For this review, take the finished solid that the model builds, in its own axes (mm). Face numbers are marked on the shaded views. A direction names the side the tool comes from. Coordinates: 2 decimals unless noted, no trailing zeros. Loops run counter-clockwise (first coordinate to the right, second up) from the corner with the lowest first, then second, coordinate; pieces in that order, holes last. Notation, with made-up numbers: M -16.75,-28 L 40.25,-28 A9 cw 40.25,-21 Z; hole C 1,73.25 d11. An arc over 180 degrees is marked long. Answer as a JSON object with one key per item and string values. Group by question number.
Item 1: Wall thickness on L1, parallel to Y at x = 0.5, z = 9; L2, parallel to Z at x = 18, y = -1.5; L3, parallel to Y at x = 40.5, z = 4.5: over which ranges is each line inside the solid? List them lowest first. Write a range as from..to.
Item 2: Mouldability with a two-part tool opening along X and no side actions: class the marked faces 1, 2 and 3 as +X half, -X half, draft (parallel to the pull), parting line (faces both ways), or undercut.
Item 3: Add section A-A (y = 0). Count the separate pieces of the cut face and the enclosed holes in it, then the cut area to 3 significant figures.
Item 4: Add section D-D (x = 37.5). State the section outline as (y, z) points.
Item 5: Insertion check: pin 1 (3 mm diameter, centred on x = 29.16, y = -29.16, fed in from -Z); pin 2 (2 mm diameter, centred on x = 29.16, y = 29.16, fed in from -Z); pin 3 (1 mm diameter, centred on x = -12.5, z = 2.5, fed in from +Y); pin 4 (3 mm diameter, centred on x = 19.5, z = 9, fed in from +Y). Each pin has a flat end and moves straight along its axis. Give the tip position at first contact, or say it passes through.
Item 6: Add section C-C (x = 3). State the section outline as (y, z) points.
Item 7: Tool access review of the marked faces 4, 5 and 6: name each direction out of +Z, -Z, +X, -X, +Y, -Y from which nothing blocks a thin tool from reaching the whole face with its end or side.
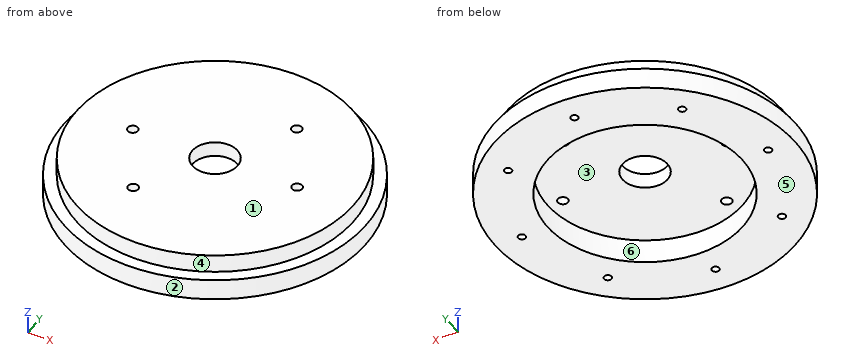
Autodesk Inventor part; units mm, degrees
ref_plane "Work Plane1" through (0, 0, 22) normal (0, 0, 1) x (1, 0, 0)
ref_plane "Plano de trabajo2" through (0, 0, 54) normal (0, 0, 1) x (1, 0, 0)
ref_plane "YZ Plane" through (0, 0, 0) normal (1, 0, 0) x (0, 1, 0)
sketch "Sketch1" plane through (0, 0, 0) normal (0, 0, 1) x (1, 0, 0)
  circle A0 centre (0, 0) radius 50
  circle A1 centre (0, 0) radius 12.5
  circle A2 centre (0, 0) radius 14.5
  line L0 (-15.5, -15.5) -> (15.5, -15.5) construction
  line L1 (15.5, -15.5) -> (15.5, 15.5) construction
  line L2 (15.5, 15.5) -> (-15.5, 15.5) construction
  line L3 (-15.5, 15.5) -> (-15.5, -15.5) construction
  line L4 (-15.5, -15.5) -> (15.5, 15.5) construction
  line L5 (15.5, -15.5) -> (-15.5, 15.5) construction
  dimension "Diametro" = 100
  dimension "d1" = 25
  dimension "d2" = 2
  dimension "d8" = 31
extrude "Extrusion1" add sketch "Sketch1" along normal blind 7 contours A0 | A2
extrude "Extrusion2" add sketch "Sketch1" along normal blind 100 contours A2
ref_plane "Work Plane1" through (0, 0, 22) normal (0, 0, 1) x (1, 0, 0)
sketch "Sketch2" plane through (0, 0, 22) normal (0, 0, 1) x (1, 0, 0)
  arc A0 (2.5, 24.8747) -> (-2.5, 24.8747) centre (0, 0) ccw
  line L0 (2.5, 24.8747) -> (2.5, 14.2829)
  line L1 (-2.5, 24.8747) -> (-2.5, 14.2829)
  line L2 (0, -70) -> (0, 70)
  circle A1 centre (0, 0) radius 14.5
  point P0 (0, 25)
  dimension "d24" = 5
  dimension "d25" = 25
  dimension "Dedos" = 5
extrude "Extrusion3" add sketch "Sketch2" along normal blind 15 contours L0 A1 L2 A0 | L2 A1 L1 A0
sketch "Sketch3" plane through (0, 0, 0) normal (1, 0, 0) x (0, 1, 0)
  line L0 (25, 37) -> (24.8747, 37)
  line L1 (14.2829, 22) -> (14.5, 22)
  line L2 (25, 22) -> (25, 37)
  line L3 (14.2829, 22) -> (14.2829, 37)
  circle A0 centre (25.74, 29.5) radius 1.5
  line L4 (0, -7.4) -> (0, 44.4)
  point P0 (0, 0)
  point P1 (25, 29.5)
  dimension "d31" = 3
  dimension "d92" = 25.74
fillet "Fillet2" radius 8 1 edges at (0, 25, 22)
pattern_circular "Circular Pattern1" count 4 over 360 about axis through (0, 0, 0) along (0, 0, 1) of "Fillet2", "Extrusion3"
ref_plane "Plano de trabajo2" through (0, 0, 54) normal (0, 0, 1) x (1, 0, 0)
sketch "Boceto4" plane through (0, 0, 54) normal (0, 0, 1) x (1, 0, 0)
  circle A0 centre (0, 0) radius 17.5
  circle A1 centre (0, 0) radius 14.5
  line L0 (4, -23.75) -> (4, -26.75)
  dimension "d54" = 35
extrude "Extrusión5" add sketch "Boceto4" against normal up to surface (47 mm away)
sketch "Boceto5" plane through (0, 0, 37) normal (0, 0, 1) x (0, 1, 0)
  arc A0 (-2.5, -17.3205) -> (2.5, -17.3205) centre (0, 0) ccw
  line L0 (-2.5, -17.3205) -> (-2.5, -24.8747)
  arc A1 (-2.5, -24.8747) -> (2.5, -24.8747) centre (0, 0) ccw
  line L1 (2.5, -24.8747) -> (2.5, -17.3205)
  circle A2 centre (0, 0) radius 14.5
  line L2 (2.5, -17.3205) -> (2.5, -14.2829)
  line L3 (-2.5, -17.3205) -> (-2.5, -14.2829)
extrude "Extrusión6" add sketch "Boceto5" along normal blind 20 contours L3 A2 L2 A0 | A0 L1 A1 L0
fillet "Empalme4" radius 8 1 edges at (25, 0, 57)
pattern_circular "Patrón circular2" count 4 over 360 about axis through (0, 0, 54) along (0, 0, -1) of "Extrusión6", "Empalme4"
chamfer "Chaflán1" distance 2 angle 45 1 edges at (-14.5, 0, 100)
sketch "Boceto6" plane through (0, 0, 7) normal (0, 0, 1) x (1, 0, 0)
  circle A0 centre (0, 0) radius 50
  arc A1 (17.3205, 2.5) -> (2.5, 17.3205) centre (0, 0) ccw construction
  line L0 (0, 0) -> (32.476, 18.75) construction
  arc A2 (17.3205, 2.5) -> (2.5, 17.3205) centre (0, 0) ccw construction
  point P0 (16.25, -6.4952)
  point P1 (16.25, 6.4952)
  point P2 (0, 37.5)
  point P3 (-32.476, 18.75)
  point P4 (-32.476, -18.75)
  point P5 (0, -37.5)
  point P6 (32.476, -18.75)
  point P7 (10.8253, 13.75)
  point P8 (15.1554, 8.75)
  dimension "d73" = 360
  dimension "d91" = 37.5
sketch "Boceto8" plane through (0, 0, 7) normal (0, 0, 1) x (1, 0, 0)
  circle A0 centre (0, 0) radius 17.5
  circle A1 centre (0, 0) radius 50
  circle A2 centre (0, 0) radius 46
  dimension "Espesor" = 4
extrude "Extrusión8" add sketch "Boceto8" along normal blind 6 contours A2
sketch "Boceto9" plane through (2.5, 14.0104, 54) normal (1, 0, 0) x (0, -1, 0)
  line L0 (16.5104, 0) -> (28.2932, 0)
  line L1 (-35.9896, 54) -> (64.0104, 54)
  point P0 (1.4018, 24.5)
  point P1 (22.4018, 0)
  dimension "d124" = 21
  dimension "d125" = 29.5
hole "Agujero4" at (2.5, 12.6086, 29.5) direction (-1, 0, 0) diameter 3.4 depth 5
pattern_circular "Patrón circular3" count 4 over 360 about axis through (0, 0, 54) along (0, 0, -1) of "Agujero4"
sketch "Boceto13" plane through (0, 0, 13) normal (0, 0, 1) x (1, 0, 0)
  point P0 (0, 0)
sketch "Boceto15" plane through (0, 0, 0) normal (0, 0, -1) x (-1, 0, 0)
  circle A0 centre (0, 0) radius 27.5 construction
  point P0 (27.5, 0)
  point P1 (13.75, 23.8157)
  point P2 (-13.75, 23.8157)
  point P3 (-27.5, 0)
  point P4 (-13.75, -23.8157)
  point P5 (13.75, -23.8157)
  dimension "d134" = 55
  dimension "d137" = 360
hole "Agujero8" at (-13.75, -23.8157, 0) at (13.75, -23.8157, 0) at (27.5, 0, 0) at (13.75, 23.8157, 0) at (-13.75, 23.8157, 0) at (-27.5, 0, 0) direction (0, 0, 1) diameter 3.4 end through all
sketch "Boceto16" plane through (0, 0, 0) normal (0, 0, -1) x (-1, 0, 0)
  circle A0 centre (0, 0) radius 32.465
  dimension "d146" = 64.93
extrude "Extrusión10" cut sketch "Boceto16" against normal blind 8
sketch "Boceto18" plane through (0, 0, 0) normal (0, 0, -1) x (-1, 0, 0)
  point P0 (0, 0)
  point P1 (-41.233, 0)
  point P2 (-29.1561, -29.1561)
  point P3 (0, -41.233)
  point P4 (29.1561, -29.1561)
  point P5 (41.233, 0)
  point P6 (29.1561, 29.1561)
  point P7 (0, 41.233)
  point P8 (-29.1561, 29.1561)
  dimension "d162" = 41.233
  dimension "d165" = 360
hole "Agujero10" at (41.233, 0, 0) at (29.1561, -29.1561, 0) at (0, -41.233, 0) at (-29.1561, -29.1561, 0) at (-41.233, 0, 0) at (-29.1561, 29.1561, 0) at (0, 41.233, 0) at (29.1561, 29.1561, 0) direction (0, 0, 1) diameter 2.459 depth 10
sketch "Sketch19" plane through (14.2829, -2.5, 54) normal (0, -1, 0) x (1, 0, 0)
  circle A0 centre (6.7167, -24.5) radius 1.7
  line L0 (3.0377, 0) -> (3.0377, -31.9844)
  line L1 (3.0377, 0) -> (-11.7829, 0)
  point P0 (-14.2829, -54)
  dimension "d174" = 3.4
  dimension "d175" = 3.679
  dimension "d176" = 24.5
hole "Hole11" at (20.9995, -2.5, 29.5) direction (0, 1, 0) diameter 4 depth 5
pattern_circular "Circular Pattern4" count 4 over 360 about axis through (0, 0, 0) along (0, 0, 1) of "Hole11"
sketch "Sketch20" plane through (0, 0, 13) normal (0, 0, 1) x (1, 0, 0)
  circle A0 centre (-27.5, 0) radius 1.7
  circle A1 centre (-13.75, 23.8157) radius 1.7
  circle A2 centre (13.75, 23.8157) radius 1.7
  circle A3 centre (27.5, 0) radius 1.7
  circle A4 centre (13.75, -23.8157) radius 1.7
  circle A5 centre (-13.75, -23.8157) radius 1.7
  circle A6 centre (0, 0) radius 46
  circle A7 centre (0, 0) radius 17.5
  circle A8 centre (0, 0) radius 46
extrude "Extrusion12" cut sketch "Sketch20" along normal up to surface contours A6 | A7
sketch "Sketch21" plane through (0, 0, 13) normal (0, 0, 1) x (1, 0, 0)
  circle A0 centre (0, 0) radius 12.5
  circle A1 centre (-27.5, 0) radius 1.7
  circle A2 centre (-13.75, 23.8157) radius 1.7
  circle A3 centre (13.75, 23.8157) radius 1.7
  circle A4 centre (27.5, 0) radius 1.7
  circle A5 centre (13.75, -23.8157) radius 1.7
  circle A6 centre (-13.75, -23.8157) radius 1.7
  circle A7 centre (0, 0) radius 46
  circle A8 centre (-13.75, 23.8157) radius 1.7
  circle A9 centre (13.75, -23.8157) radius 1.7
extrude "Extrusion13" add sketch "Sketch21" against normal up to surface (5 mm away) contours A2 | A5
sketch "Sketch23" plane through (0, 0, 13) normal (0, 0, 1) x (1, 0, 0)
  circle A0 centre (0, 0) radius 12.5
  circle A1 centre (-27.5, 0) radius 1.7
  circle A2 centre (13.75, 23.8157) radius 1.7
  circle A3 centre (27.5, 0) radius 1.7
  circle A4 centre (-13.75, -23.8157) radius 1.7
  circle A5 centre (0, 0) radius 46
  circle A6 centre (0, 0) radius 7.5
  dimension "d192" = 15
extrude "Extrusion14" add sketch "Sketch23" against normal up to surface (5 mm away) contours A0
equation "\"d24\" = Dedos"
equation "\"d91\" = 0.375 * Diametro"
properties part number "Soporte22" material "Aluminum 7075"
From the geometry:
{
 "1": {"L1": "y = -46..-42.36, -40.11..-7.48, 7.48..40.11, 42.36..46", "L2": "z = 8..13", "L3": "y = -29.32..-0.99, 0.99..29.32"},
 "2": {"face 1": "draft", "face 2": "parting line", "face 3": "undercut"},
 "3": {"separate pieces": "4", "enclosed holes": "0", "area": "574 mm²"},
 "4": {"outline": "M -33.07,0 L 33.07,0 L 33.07,7 L 26.64,7 L 26.64,13 L -26.64,13 L -26.64,7 L -33.07,7 Z"},
 "5": {"pin 1": "stops at z = 0", "pin 2": "stops at z = 10", "pin 3": "stops at y = 48.54", "pin 4": "stops at y = 42.33"},
 "6": {"outline": "M -49.91,0 L -32.33,0 L -32.33,8 L -6.87,8 L -6.87,13 L -45.9,13 L -45.9,7 L -49.91,7 Z; M 6.87,8 L 32.33,8 L 32.33,0 L 49.91,0 L 49.91,7 L 45.9,7 L 45.9,13 L 6.87,13 Z"},
 "7": {"face 4": "+Z", "face 5": "-Z, +X, -X, +Y, -Y", "face 6": "-Z"}
}
